from build123d import *

# Parameters (mm, degrees)
SKETCH1_R           = 48
BOSS_EXTRUDE1_DEPTH = 3
SKETCH2_R           = 1.75
CUT_EXTRUDE1_DEPTH  = 3
CIRPATTERN1_COUNT   = 6
SKETCH3_R           = 8
BOSS_EXTRUDE2_DEPTH = 53
SKETCH4_R           = 3.2
CUT_EXTRUDE2_DEPTH  = 89
CHAMFER1_SIZE       = 1
FILLET1_SIZE        = 8
SKETCH5_R           = 19.25
BOSS_EXTRUDE3_DEPTH = 3


with BuildPart() as part:
    # Sketch1 → Boss-Extrude1 (new body)
    with BuildSketch(Plane.XY):
        Circle(SKETCH1_R)
    extrude(amount=BOSS_EXTRUDE1_DEPTH)

    # Sketch2 → Cut-Extrude1 (cut)
    with BuildSketch(Plane.XY.offset(3)):
        with Locations((0, 40)):
            Circle(SKETCH2_R)
    cut_extrude1 = extrude(amount=-CUT_EXTRUDE1_DEPTH, mode=Mode.SUBTRACT)

    # CirPattern1: Cut-Extrude1 ×6 about axis
    cirpattern1_axis = Axis((0, 0, 0), (0, 0, 1))
    for i in range(1, CIRPATTERN1_COUNT):
        add(cut_extrude1.rotate(cirpattern1_axis, i * 360 / CIRPATTERN1_COUNT), mode=Mode.SUBTRACT)

    # Sketch3 → Boss-Extrude2 (add)
    with BuildSketch(Plane.XY.offset(3)):
        with Locations((24.5, 0)):
            Circle(SKETCH3_R)
    extrude(amount=BOSS_EXTRUDE2_DEPTH)

    # Sketch4 → Cut-Extrude2 (cut, through all)
    with BuildSketch(Plane.XY.offset(56)):
        with Locations((24.5, 0)):
            Circle(SKETCH4_R)
    extrude(amount=-CUT_EXTRUDE2_DEPTH, mode=Mode.SUBTRACT)

    # Chamfer1
    chamfer1_edges = [part.edges().sort_by_distance(p)[0] for p in [
        (21.3, 0, 56),
    ]]
    chamfer(chamfer1_edges, length=CHAMFER1_SIZE)

    # Fillet1
    # a fillet whose section is not a circle: 8 mm, written as the material it adds along each edge
    with BuildSketch(Plane(origin=(24.5, 0, 3), x_dir=(1, 0, 0), z_dir=(0, -1, 0))) as fillet1_piece_1:
        with BuildLine():
            Bezier((8, FILLET1_SIZE), (8, 0), (8 + FILLET1_SIZE, 0), weights=[1, 0.25, 1])
            Line((8 + FILLET1_SIZE, 0), (8, 0))
            Line((8, 0), (8, FILLET1_SIZE))
        make_face()
    revolve(axis=Axis((24.5, 0, 3), (0, 0, 1)))

    # Sketch5 → Boss-Extrude3 (add)
    with BuildSketch(Plane.XY.offset(3)):
        Circle(SKETCH5_R)
    extrude(amount=BOSS_EXTRUDE3_DEPTH)


solid = part.part
Check sheet for the modelled part. Datum: model origin and axes. Units: mm. A direction names the side the tool comes from. Coordinates: 2 decimals unless noted, no trailing zeros. Loops run counter-clockwise (first coordinate to the right, second up) from the corner with the lowest first, then second, coordinate; pieces in that order, holes last. Notation, with made-up numbers: (-16, 72.25) -> (-2, 72.25) arc R37 cw to (-2, 109.25) -> close; hole circle Ø11 at (-24, -12.5). An arc over 180 degrees is marked (long way). Write item = value, one per line. Start each with the question number.
1. Draft check along X on faces 1 (the cylindrical face through (21.3, 0.1, 27.9)), 2 (the cylindrical face through (18.151, -4.868, 33.185)), 3 (the flat face through (-1, 1, 0)). Enter one of: released by +X, released by -X, zero draft, split by the parting line, or undercut.
2. Section check D-D on y = -30. Record the cut outline in (x, z).
3. Section check A-A on y = -40. Record the cut outline in (x, z), then the cut area to 3 significant figures.
4. Tool access check on faces 4 (the cylindrical face through (-35.931, -18.817, 1.521)), 5 (the cylindrical face through (-19.237, 0.72, 4.479)). Record the directions out of +Z, -Z, +X, -X, +Y, -Y that give a thin tool (end or side, any length) a straight path to the whole face; none if there is none.
5. Depth check by flat-ended pin: P1, Ø3, axis at x = 34.64, y = -20, coming from the +Z side; P2, Ø4.5, axis at x = -34.64, y = 20, coming from the +Z side; P3, Ø4, axis at y = -6.5, z = 18, coming from the +X side; P4, Ø18, axis at x = 4, y = -2.5, coming from the +Z side. Enter the tip coordinate at first touch or a pass-through.
6. Material ranges on line 1 (Y direction, x = 0, z = 0.8); line 2 (Z direction, x = -27.5, y = -21); line 3 (Y direction, x = 22, z = 6), recorded low to high.
7. Section check B-B on x = 11.5. Record the cut outline in (y, z), then the cut area to 3 significant figures.
8. Section check C-C on z = 27.5. Record the cut outline in (x, y), then the cut area to 3 significant figures.
Responses:
q1.face_1 = undercut
q1.face_2 = split by the parting line
q1.face_3 = zero draft
q2.outline = (-37.47, 0) -> (37.47, 0) -> (37.47, 3) -> (-37.47, 3) -> close
q3.outline = (-26.53, 0) -> (-1.75, 0) -> (-1.75, 3) -> (-26.53, 3) -> close; (1.75, 0) -> (26.53, 0) -> (26.53, 3) -> (1.75, 3) -> close
q3.area = 149 mm2
q4.face_4 = +Z, -Z
q4.face_5 = +Z
q5.P1 = through
q5.P2 = 3
q5.P3 = 31.11
q5.P4 = 6
q6.line_1 = -48 to -41.75, -38.25 to 38.25, 41.75 to 48
q6.line_2 = 0 to 3
q6.line_3 = -11.13 to -2, 2 to 11.13
q7.outline = (-46.6, 0) -> (46.6, 0) -> (46.6, 3) -> (15.44, 3) -> (15.44, 6) -> (-15.44, 6) -> (-15.44, 3) -> (-46.6, 3) -> close
q7.area = 372 mm2
q8.outline = circle Ø16 at (24.5, 0); hole circle Ø6.4 at (24.5, 0)
q8.area = 169 mm2
